from build123d import *

# Parameters (mm, degrees)
SKETCH2_R               = 60.325
SKETCH2_R_2             = 3.96875
SKETCH2_R_3             = 12.7
BOSS_EXTRUDE1_DEPTH     = 19.05
SKETCH3_R               = 73.025
SKETCH3_R_2             = 3.96875
SKETCH3_R_3             = 12.7
BOSS_EXTRUDE2_DEPTH     = 3.175
BOSS_EXTRUDE3_START     = 3.175
SKETCH4_R               = 73.025
SKETCH4_R_2             = 12.7
SKETCH4_R_3             = 3.96875
BOSS_EXTRUDE3_DEPTH     = 3.175
CUT_EXTRUDE1_DEPTH      = 106.637360224
CUT_EXTRUDE1_DEPTH_BACK = 106.637360224


with BuildPart() as part:
    # Sketch2 → Boss-Extrude1 (new body)
    with BuildSketch(Plane(origin=(0, 0, 0), x_dir=(1, 0, 0), z_dir=(0, 1, 0))):
        with Locations(Location((0, 0, 0), (0, 0, 90))):
            Circle(SKETCH2_R)
        with Locations(Location((0, 25.4, 0), (0, 0, 90))):
            Circle(SKETCH2_R_2, mode=Mode.SUBTRACT)
        with Locations(Location((21.997045256, 12.7, 0), (0, 0, 90))):
            Circle(SKETCH2_R_2, mode=Mode.SUBTRACT)
        with Locations(Location((21.997045256, -12.7, 0), (0, 0, 90))):
            Circle(SKETCH2_R_2, mode=Mode.SUBTRACT)
        with Locations(Location((0, -25.4, 0), (0, 0, 90))):
            Circle(SKETCH2_R_2, mode=Mode.SUBTRACT)
        with Locations(Location((-21.997045256, -12.7, 0), (0, 0, 90))):
            Circle(SKETCH2_R_2, mode=Mode.SUBTRACT)
        with Locations(Location((-21.997045256, 12.7, 0), (0, 0, 90))):
            Circle(SKETCH2_R_2, mode=Mode.SUBTRACT)
        with Locations(Location((0, 0, 0), (0, 0, 90))):
            Circle(SKETCH2_R_3, mode=Mode.SUBTRACT)
    extrude(amount=BOSS_EXTRUDE1_DEPTH)

    # Sketch3 → Boss-Extrude2 (add)
    with BuildSketch(Plane(origin=(0, 19.05, 0), x_dir=(1, 0, 0), z_dir=(0, 1, 0))):
        with Locations(Location((0, 0, 0), (0, 0, 270))):
            Circle(SKETCH3_R)
        with Locations(Location((0, 25.4, 0), (0, 0, 90))):
            Circle(SKETCH3_R_2, mode=Mode.SUBTRACT)
        with Locations(Location((21.997045256, 12.7, 0), (0, 0, 90))):
            Circle(SKETCH3_R_2, mode=Mode.SUBTRACT)
        with Locations(Location((21.997045256, -12.7, 0), (0, 0, 90))):
            Circle(SKETCH3_R_2, mode=Mode.SUBTRACT)
        with Locations(Location((0, -25.4, 0), (0, 0, 90))):
            Circle(SKETCH3_R_2, mode=Mode.SUBTRACT)
        with Locations(Location((-21.997045256, -12.7, 0), (0, 0, 90))):
            Circle(SKETCH3_R_2, mode=Mode.SUBTRACT)
        with Locations(Location((0, 0, 0), (0, 0, 90))):
            Circle(SKETCH3_R_3, mode=Mode.SUBTRACT)
        with Locations(Location((-21.997045256, 12.7, 0), (0, 0, 90))):
            Circle(SKETCH3_R_2, mode=Mode.SUBTRACT)
    extrude(amount=BOSS_EXTRUDE2_DEPTH)

    # Sketch4 → Boss-Extrude3 (add)
    with BuildSketch(Plane.XZ.offset(BOSS_EXTRUDE3_START)):
        with Locations(Location((0, 0, 0), (0, 0, 90))):
            Circle(SKETCH4_R)
        with Locations(Location((0, 0, 0), (0, 0, 270))):
            Circle(SKETCH4_R_2, mode=Mode.SUBTRACT)
        with Locations(Location((-21.997045256, -12.7, 0), (0, 0, 270))):
            Circle(SKETCH4_R_3, mode=Mode.SUBTRACT)
        with Locations(Location((0, -25.4, 0), (0, 0, 270))):
            Circle(SKETCH4_R_3, mode=Mode.SUBTRACT)
        with Locations(Location((21.997045256, -12.7, 0), (0, 0, 270))):
            Circle(SKETCH4_R_3, mode=Mode.SUBTRACT)
        with Locations(Location((21.997045256, 12.7, 0), (0, 0, 270))):
            Circle(SKETCH4_R_3, mode=Mode.SUBTRACT)
        with Locations(Location((0, 25.4, 0), (0, 0, 270))):
            Circle(SKETCH4_R_3, mode=Mode.SUBTRACT)
        with Locations(Location((-21.997045256, 12.7, 0), (0, 0, 270))):
            Circle(SKETCH4_R_3, mode=Mode.SUBTRACT)
    extrude(amount=-BOSS_EXTRUDE3_DEPTH)

    # Sketch6 → Cut-Extrude1 (cut, two sides: drawn at the far end of the back side and taken through both)
    with BuildSketch(Plane(origin=(0, 0, 0), x_dir=(1, 0, 0), z_dir=(0, 1, 0)).offset(-CUT_EXTRUDE1_DEPTH_BACK)):
        with BuildLine():
            ThreePointArc((21.314275493, 49.588328115), (1.249191015, 53.960542499), (-18.996723984, 50.521531082))
            Line((-18.996723984, 50.521531082), (-11.255118383, 33.061729162))
            ThreePointArc((-11.255118383, 33.061729162), (0.178151467, 34.924545624), (11.591822226, 32.945186029))
            Line((11.591822226, 32.945186029), (21.314275493, 49.588328115))
        make_face()
        with BuildLine():
            ThreePointArc((-31.283856312, 43.984326291), (-46.343943604, 27.668384778), (-53.561272173, 6.670138541))
            Line((-53.561272173, 6.670138541), (-34.259856576, 6.783645952))
            ThreePointArc((-34.259856576, 6.783645952), (-30.348105608, 17.284331372), (-23.312207546, 26.005703304))
            Line((-23.312207546, 26.005703304), (-31.283856312, 43.984326291))
        make_face()
        with BuildLine():
            ThreePointArc((-53.47911905, -7.299619899), (-46.638038937, -27.169724863), (-32.727191245, -42.921225264))
            Line((-32.727191245, -42.921225264), (-23.004737979, -26.278083178))
            ThreePointArc((-23.004737979, -26.278083178), (-30.1427228, -17.640064829), (-34.177703438, -7.186112487))
            Line((-34.177703438, -7.186112487), (-53.47911905, -7.299619899))
        make_face()
        with BuildLine():
            Line((-11.591822226, -32.945186029), (-21.314275493, -49.588328115))
            ThreePointArc((-21.314275493, -49.588328115), (0.938377322, -53.966842348), (23.025356811, -48.817349054))
            Line((23.025356811, -48.817349054), (11.255118563, -33.061729101))
            ThreePointArc((11.255118563, -33.061729101), (-0.178151371, -34.924545625), (-11.591822226, -32.945186029))
        make_face()
        with BuildLine():
            Line((23.312207688, -26.005703177), (34.742784352, -41.306652739))
            ThreePointArc((34.742784352, -41.306652739), (47.427034742, -25.767751175), (53.56127215, -6.670138728))
            Line((53.56127215, -6.670138728), (34.259856539, -6.783646139))
            ThreePointArc((34.259856539, -6.783646139), (30.348105608, -17.284331372), (23.312207688, -26.005703177))
        make_face()
        with BuildLine():
            Line((34.177703478, 7.186112301), (53.479119075, 7.299619712))
            ThreePointArc((53.479119075, 7.299619712), (46.638038984, 27.169724781), (32.727191245, 42.921225264))
            Line((32.727191245, 42.921225264), (23.004737979, 26.278083178))
            ThreePointArc((23.004737979, 26.278083178), (30.142722848, 17.640064747), (34.177703478, 7.186112301))
        make_face()
    extrude(amount=CUT_EXTRUDE1_DEPTH + CUT_EXTRUDE1_DEPTH_BACK, mode=Mode.SUBTRACT)


solid = part.part
Model file for the job. Use its own axes, mm. A direction names the side the tool comes from. Give positions to 0.01 mm unless a question says otherwise; leave off trailing zeros. Order: outer loops, then holes, each group sorted by start corner. A loop starts at its lowest first (then second) coordinate and runs counter-clockwise, first axis right, second up. Notation, with made-up numbers: (41.25, -10.75) - (57.25, -10.75) arc R14 ccw to (57.25, 9.25) - close; hole circle Ø1 at (-23, 30.5). An arc over 180 degrees is marked (long way). Return JSON: item names as keys, results as strings.
1) Cut at A-A, the plane z = 0. Give the cut face in (x, y) (3 decimals), plus the area to 3 significant figures.
Geometry says:
{"outline": "(-73.025, -3.175) - (-12.7, -3.175) - (-12.7, 22.225) - (-73.025, 22.225) - (-73.025, 19.05) - (-60.325, 19.05) - (-60.325, 0) - (-73.025, 0) - close; (12.7, -3.175) - (73.025, -3.175) - (73.025, 0) - (60.325, 0) - (60.325, 19.05) - (73.025, 19.05) - (73.025, 22.225) - (12.7, 22.225) - close", "area": "2,580 mm²"}
2) Cut at C-C, the plane y = 16.25. Count the separate pieces of the cut face and the enclosed holes in it, plus the area to 3 significant figures.
Geometry says:
{"separate pieces": "1", "enclosed holes": "13", "area": "6,880 mm²"}
3) Probe line 1 (X direction, y = 10.5, z = -23); line 2 (Y direction, x = 49, z = -45.5) (3 decimals); line 3 (Z direction, x = 3, y = 3.25). List the from-to ranges inside material, lowest first. Write a range as from..to.
Geometry says:
{"line 1": "-55.77..-48.83, -26.28..-3.16, 3.16..26.28, 48.83..55.77", "line 2": "-3.175..0, 19.05..22.225", "line 3": "-60.25..-53.89, -34.8..-28, -22.8..-12.34, 12.34..22.8, 28..34.8, 53.89..60.25"}
4) Pull direction X, two halves, no side cores. Call faces 1 (the cylindrical face through (-30.06, 9.35, 17.78)), 2 (the cylindrical face through (0.62, 9.35, 53.97)), 3 (the flat face through (60, 19.05, 10)), 4 (the cylindrical face through (-21.935, -1.61, 69.653)): pulls with the +X half, pulls with the -X half, needs draft (parallel to the pull), parting line crosses it, or undercut.
Geometry says:
{"face 1": "undercut", "face 2": "undercut", "face 3": "needs draft", "face 4": "parting line crosses it"}
5) Cut at B-B, the plane x = -63.5. Give the cut face in (y, z) (3 decimals).
Geometry says:
{"outline": "(-3.175, -36.061) - (0, -36.061) - (0, 36.061) - (-3.175, 36.061) - close; (19.05, -36.061) - (22.225, -36.061) - (22.225, 36.061) - (19.05, 36.061) - close"}
6) Flat gauge pins, fed straight in: P1, Ø10, axis at x = -46, y = 17.5, coming from the +Z side; P2, Ø2, axis at x = 16, y = 2.5, coming from the -Z side; P3, Ø10, axis at y = 6.5, z = -57.5, coming from the +X side; P4, Ø12.5, axis at x = 0, z = 25.4, coming from the -Y side (3 decimals). Where does each tip first touch, or does it go through?
Geometry says:
{"P1": "z = 60.26", "P2": "z = -58.43", "P3": "x = 29.71", "P4": "y = -3.175"}
7) 3-axis set-ups, long thin cutter, end or side, ignore diameter. For faces 5 (the flat face through (-15, 22.225, -1)), 6 (the cylindrical face through (30.426, 9.347, 17.147)), 7 (the cylindrical face through (-2.652, 9.392, 60.267)): which of +Z, -Z, +X, -X, +Y, -Y reach the whole face in a straight line?
Geometry says:
{"face 5": "+Z, -Z, +X, -X, +Y", "face 6": "+Y, -Y", "face 7": "none"}
8) Cut at D-D, the plane x = 46. Give the cut face in (y, z) (3 decimals).
Geometry says:
{"outline": "(-3.175, -56.716) - (0, -56.716) - (0, -39.027) - (19.05, -39.027) - (19.05, -56.716) - (22.225, -56.716) - (22.225, -28.237) - (-3.175, -28.237) - close; (-3.175, -7.256) - (22.225, -7.256) - (22.225, 6.715) - (-3.175, 6.715) - close; (-3.175, 28.237) - (22.225, 28.237) - (22.225, 56.716) - (19.05, 56.716) - (19.05, 39.027) - (0, 39.027) - (0, 56.716) - (-3.175, 56.716) - close"}
